Verification items for the finished model (mm, model axes). A direction names the side the tool comes from. Give positions to 0.01 mm unless a question says otherwise; leave off trailing zeros. Write each loop counter-clockwise with the first axis right and the second up, starting at its lowest first coordinate (ties: lowest second). Pieces come first, ordered by that corner, then holes. Notation, with made-up numbers: (62.25, 58) -> (104.25, 58) arc R10 cw to (104.25, 73) -> close; hole circle Ø6 at (10.25, -19.75). An arc over 180 degrees is marked (long way). Answer as CSV lines item,"result".
```python
from build123d import *

# Parameters (mm, degrees)
F3_DEPTH = 1.5875
F4_R     = 0.79375
F5_DEPTH = 3.175
F6_DEPTH = 1.5875


# Not quite as in the source:
# - a length typed as a fraction of an inch, garbled in the dataset ("3 / 203.2 mm" for 3/8 in), is restored


with BuildPart() as f3:
    # F2 (on line) → F3 (new body)
    with BuildSketch(Plane(origin=(0, 0, 55.2947693627), x_dir=(1, 0, 0), z_dir=(0, 0, -1))):
        with BuildLine():
            ThreePointArc((9.525, 0), (0, 9.525), (-9.525, 0))
            Line((-9.525, 0), (-9.525, -9.525))
            Line((-9.525, -9.525), (9.525, -9.525))
            Line((9.525, -9.525), (9.525, 0))
        make_face()
    extrude(amount=-F3_DEPTH)

    # F4 (on Right) → F5 (join, symmetric)
    with BuildSketch(Plane.YZ):
        with BuildLine():
            Line((9.525, 42.5947693627), (9.525, 55.2947693627))
            Line((9.525, 55.2947693627), (6.985, 55.2947693627))
            Line((6.985, 55.2947693627), (6.985, 40.0547693627))
            ThreePointArc((6.985, 40.0547693627), (7.7289487758, 41.8508205869), (9.525, 42.5947693627))
        make_face()
        Polygon((10.16, -10.7452306373), (6.985, -10.7452306373), (6.985, -13.9202306373), (10.16, -13.9202306373), (10.16, -15.5077306373), (14.9225, -15.5077306373), (14.9225, -9.1577306373), (10.16, -9.1577306373), align=None)
        with BuildLine():
            ThreePointArc((10.3640900788, 37.6573691375), (8.0552532191, 37.9831891928), (6.985, 40.0547693627))
            Line((6.985, 40.0547693627), (6.985, -10.7452306373))
            Line((6.985, -10.7452306373), (10.16, -10.7452306373))
            Line((10.16, -10.7452306373), (10.16, -9.1577306373))
            Line((10.16, -9.1577306373), (14.9225, -9.1577306373))
            Line((14.9225, -9.1577306373), (14.9225, -15.5077306373))
            Line((14.9225, -15.5077306373), (10.16, -15.5077306373))
            Line((10.16, -15.5077306373), (10.16, -13.9202306373))
            Line((10.16, -13.9202306373), (6.985, -13.9202306373))
            Line((6.985, -13.9202306373), (6.985, -61.5452306373))
            ThreePointArc((6.985, -61.5452306373), (25.2233058777, -60.0065006912), (42.9460033775, -55.433811716))
            Line((42.9460033775, -55.433811716), (10.3640900788, 37.6573691375))
        make_face()
        with BuildLine():
            ThreePointArc((12.065, 40.0547693627), (11.3210512242, 41.8508205869), (9.525, 42.5947693627))
            ThreePointArc((9.525, 42.5947693627), (7.7289487758, 41.8508205869), (6.985, 40.0547693627))
            ThreePointArc((6.985, 40.0547693627), (8.0552532191, 37.9831891928), (10.3640900788, 37.6573691375))
            ThreePointArc((10.3640900788, 37.6573691375), (11.5965801698, 38.5850225818), (12.065, 40.0547693627))
        make_face()
        with Locations((9.525, 40.0547693627)):
            Circle(F4_R, mode=Mode.SUBTRACT)
    extrude(amount=F5_DEPTH, both=True)

    # F4 (on Right) → F6 (cut, symmetric)
    with BuildSketch(Plane.YZ):
        Polygon((10.16, -10.7452306373), (6.985, -10.7452306373), (6.985, -13.9202306373), (10.16, -13.9202306373), (10.16, -15.5077306373), (14.9225, -15.5077306373), (14.9225, -9.1577306373), (10.16, -9.1577306373), align=None)
    extrude(amount=F6_DEPTH, both=True, mode=Mode.SUBTRACT)


solid = f3.part
```
1) Tool access check on faces 4 (the flat face through (0, 9.525, 51)), 5 (the flat face through (-3.175, 21, -28)), 6 (the flat face through (0, 6.985, -2)). Record the directions out of +Z, -Z, +X, -X, +Y, -Y that give a thin tool (end or side, any length) a straight path to the whole face; none if there is none.
Reported:
face 4,"+Z, +X, -X, +Y"
face 5,"-Z, -X, +Y, -Y"
face 6,"-Z, +X, -X, -Y"
2) Draft check along Z on faces 1 (the flat face through (3.175, 21, -28)), 2 (the flat face through (0, 9, -13.92)), 3 (the flat face through (0, 0, 56.882)). Enter one of: +Z half, -Z half, draft (parallel to the pull), parting line (faces both ways), or undercut.
Reported:
face 1,"draft"
face 2,"undercut"
face 3,"+Z half"
3) Scan lines: line 1 along Z through (x, y) = (7.25, -3); line 2 along X through (y, z) = (21, -46) (3 decimals); line 3 along Y through (x, z) = (2.5, 15.5) (3 decimals). Record each from-to range of solid material in increasing order.
Reported:
line 1,"55.29 to 56.88"
line 2,"-3.175 to 3.175"
line 3,"6.985 to 18.119"
4) Section check A-A (x = 0). Record the boundary of the cut face in (y, z) (1 decimal), and give its area (3 significant figures).
Reported:
outline,"(-9.5, 55.3) -> (7, 55.3) -> (7, -10.7) -> (10.2, -10.7) -> (10.2, -9.2) -> (14.9, -9.2) -> (14.9, -15.5) -> (10.2, -15.5) -> (10.2, -13.9) -> (7, -13.9) -> (7, -61.5) arc R108.9 ccw to (42.9, -55.4) -> (10.4, 37.7) arc R2.5 ccw to (9.5, 42.6) -> (9.5, 56.9) -> (-9.5, 56.9) -> close; hole circle Ø1.6 at (9.5, 40.1)"
area,"2,020 mm²"
5) Depth check by flat-ended pin: pin 1 (1.9 mm diameter, centred on y = 11, z = -12, fed in from +X) (3 decimals); pin 2 (3 mm diameter, centred on x = -0.5, z = 23.5, fed in from -Y) (3 decimals); pin 3 (7 mm diameter, centred on y = 10, z = -11, fed in from -X) (3 decimals). Enter the tip coordinate at first touch or a pass-through.
Reported:
pin 1,"x = 3.175"
pin 2,"y = 6.985"
pin 3,"x = -3.175"
6) Section check B-B (x = 7). Record the boundary of the cut face in (y, z) (3 decimals).
Reported:
outline,"(-6.46, 55.295) -> (9.525, 55.295) -> (9.525, 56.882) -> (-6.46, 56.882) -> close"
7) Section check C-C (y = 35). Record the boundary of the cut face in (x, z) (3 decimals).
Reported:
outline,"(-3.175, -57.879) -> (3.175, -57.879) -> (3.175, -32.731) -> (-3.175, -32.731) -> close"
